Answer from the drawing. Dimensions are ordinates in mm from the lowest x, y and z of the part. A direction names the side the tool comes from. Give positions to 0.01 mm unless a question says otherwise; leave off trailing zeros. Loops run counter-clockwise (first coordinate to the right, second up) from the corner with the lowest first, then second, coordinate; pieces in that order, holes last. Notation, with made-up numbers: (62, 60.5) - (71, 60.5) arc R29 ccw to (71, 93.5) - close; hole circle Ø7 at (54, 68.5). An arc over 180 degrees is marked (long way). Answer as CSV lines item,"result". Start each with the question number.
1) Find the intervals of material crossed by line 1 along Y through (x, z) = (31, 8); line 2 along X through (y, z) = (27, 15); line 3 along X through (y, z) = (19, 20) (1 decimal), in increasing order.
2) A cutting plane is placed at D-D (z = 7). Determine the outline of the cut face in (x, y), and give its area (3 significant figures).
3) For the marked faces 1, 2 and 3, determine the directions among +Z, -Z, +X, -X, +Y, -Y from which every point of the face is accessible in a straight line to the end or side of a thin tool.
4) A cutting plane is placed at B-B (z = 12.7). Determine the outline of the cut face in (x, y) (1 decimal), and give its area (3 significant figures).
5) For a pull along X with two mould halves and no side action, classify the marked faces 4, 5, 6 and 7 as pulls with the +X half, pulls with the -X half, needs draft (parallel to the pull), parting line crosses it, or undercut.
6) Flat-ended cylindrical pins translate along their axes: pin 1 (6.5 mm diameter, centred on x = 47.5, y = 19, fed in from -Z); pin 2 (6 mm diameter, centred on x = 52.5, y = 29, fed in from +Z) (1 decimal); pin 3 (12 mm diameter, centred on y = 6, z = 32, fed in from +X). Find the tip coordinate at first contact, or state that the pin passes through.
7) A cutting plane is placed at A-A (x = 38.1). Determine the outline of the cut face in (y, z) (1 decimal), and give its area (3 significant figures).
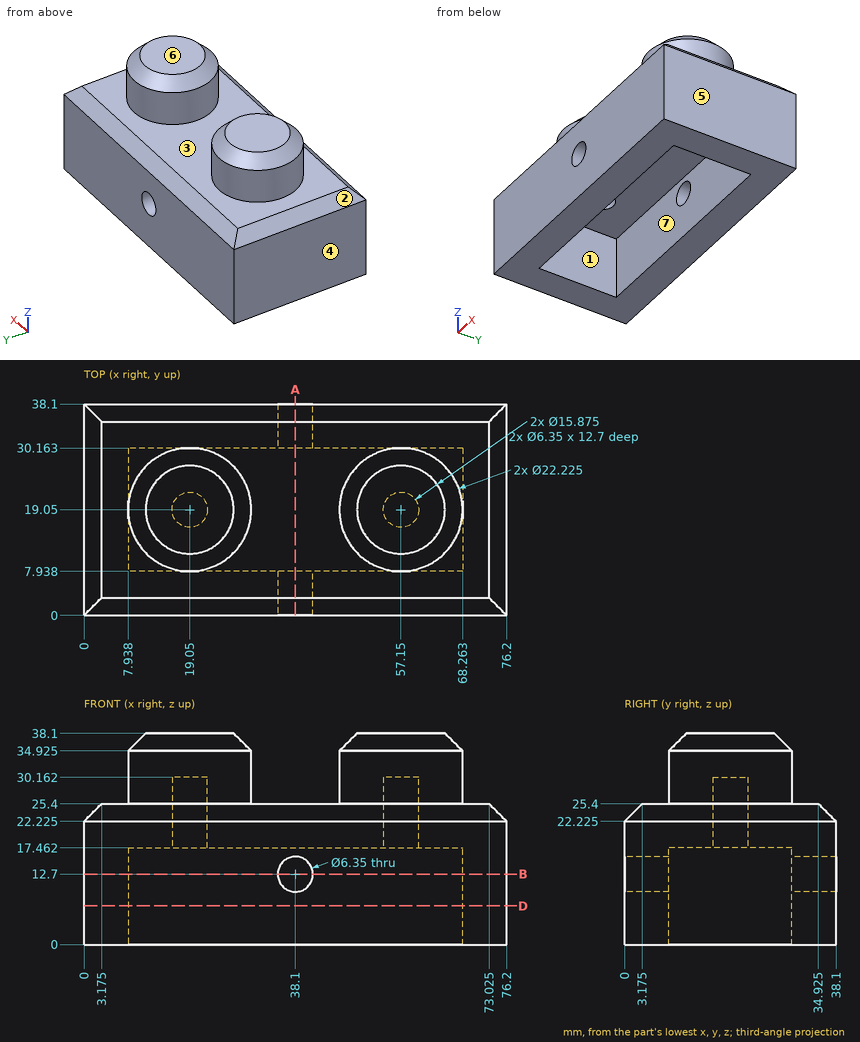
Ans:
1,line 1,"0 to 7.94, 30.16 to 38.1"
1,line 2,"0 to 7.94, 68.26 to 76.2"
1,line 3,"0 to 15.9, 22.2 to 54, 60.3 to 76.2"
2,outline,"(0, 0) - (76.2, 0) - (76.2, 38.1) - (0, 38.1) - close; hole (7.94, 7.94) - (68.26, 7.94) - (68.26, 30.16) - (7.94, 30.16) - close"
2,area,"1,560 mm2"
3,face 1,"-Z"
3,face 2,"+Z, -X, +Y, -Y"
3,face 3,"+Z"
4,outline,"(0, 0) - (34.9, 0) - (34.9, 7.9) - (7.9, 7.9) - (7.9, 30.2) - (34.9, 30.2) - (34.9, 38.1) - (0, 38.1) - close; (41.3, 0) - (76.2, 0) - (76.2, 38.1) - (41.3, 38.1) - (41.3, 30.2) - (68.3, 30.2) - (68.3, 7.9) - (41.3, 7.9) - close"
4,area,"1,460 mm2"
5,face 4,"pulls with the -X half"
5,face 5,"pulls with the +X half"
5,face 6,"needs draft"
5,face 7,"undercut"
6,pin 1,"z = 17.46"
6,pin 2,"z = 38.1"
6,pin 3,"x = 65.74"
7,outline,"(0, 0) - (7.9, 0) - (7.9, 9.5) - (0, 9.5) - close; (0, 15.9) - (7.9, 15.9) - (7.9, 17.5) - (30.2, 17.5) - (30.2, 15.9) - (38.1, 15.9) - (38.1, 22.2) - (34.9, 25.4) - (3.2, 25.4) - (0, 22.2) - close; (30.2, 0) - (38.1, 0) - (38.1, 9.5) - (30.2, 9.5) - close"
7,area,"469 mm2"
